Build history of the part. All positions in model axes, mm. Face numbers are marked on the shaded views. A direction names the side the tool comes from. Coordinates: 2 decimals unless noted, no trailing zeros. Order: outer loops, then holes, each group sorted by start corner. A loop starts at its lowest first (then second) coordinate and runs counter-clockwise, first axis right, second up. Notation, with made-up numbers: M -39.5,29.5 L 3.5,29.5 A26 ccw 3.5,65.5 Z; hole C -26,59 d8. An arc over 180 degrees is marked long. Write item = value, one per line. Start each with the question number.
Q1. Pull direction X, two halves, no side cores. Call the marked faces 1, 2 and 3: released by +X, released by -X, zero draft, split by the parting line, or undercut.
Q2. Pin check, flat tips, straight feed: P1, Ø6, axis at y = 21, z = -2.5, coming from the -X side; P2, Ø1.5, axis at x = -6, y = 21, coming from the -Z side; P3, Ø1, axis at x = -8.5, y = 16.5, coming from the +Z side. Stop position of each tip, or through.
Q3. Band-saw the part on A-A on y = 17.5. Write the cut outline in (x, z).
Q4. Drill centre lines: probe 1 along X at (y, z) = (1.3, 0); probe 2 along X at (y, z) = (20.25, 0); probe 3 along X at (y, z) = (11.5, 5). Where is each one in solid material? Low to high.
Q5. Band-saw the part on B-B on y = 6.5. Write the cut outline in (x, z).
Q6. 3-axis set-ups, long thin cutter, end or side, ignore diameter. For the marked faces 4 and 5: which of +Z, -Z, +X, -X, +Y, -Y reach the whole face in a straight line?
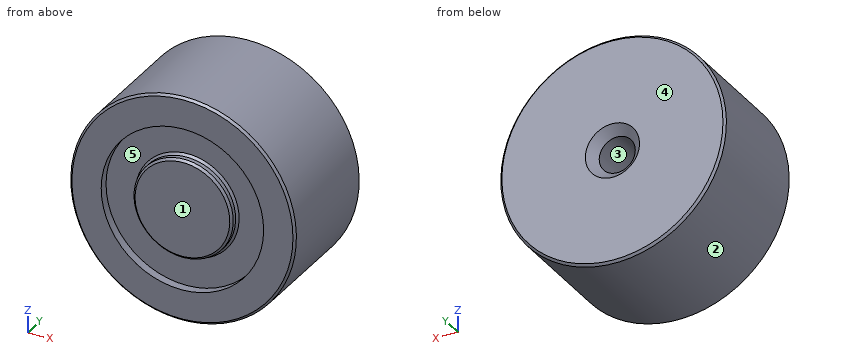
```python
from build123d import *

# Parameters (mm, degrees)
SKETCH_1_R          = 25
EXTRUDE_1_DEPTH     = 27
SKETCH_9_R          = 4
CUT_EXTRUDE_1_DEPTH = 12
CHAMFER_1_SIZE      = 2
CHAMFER_2_SIZE      = 0.5
SKETCH_11_R         = 18
SKETCH_11_R_2       = 11
CUT_EXTRUDE_2_DEPTH = 2
CHAMFER_3_SIZE      = 0.5


with BuildPart() as part:
    # 草图1 → 凸台-拉伸1 (new body)
    with BuildSketch(Plane(origin=(0, 0, 0), x_dir=(1, 0, 0), z_dir=(0, 1, 0))):
        with Locations(Location((0, 0, 0), (0, 0, 270))):
            Circle(SKETCH_1_R)
    extrude(amount=EXTRUDE_1_DEPTH)

    # 草图9 → 切除-拉伸1 (cut)
    with BuildSketch(Plane(origin=(0, 27, 0), x_dir=(1, 0, 0), z_dir=(0, 1, 0))):
        with Locations(Location((0, 0, 0), (0, 0, 270))):
            Circle(SKETCH_9_R)
    extrude(amount=-CUT_EXTRUDE_1_DEPTH, mode=Mode.SUBTRACT)

    # 草图10 → 切除-旋转2 (revolve, cut)
    with BuildSketch(Plane.XY, mode=Mode.PRIVATE) as cut_revolve_2_sk:
        Polygon((-4, 15), (0, 12.093829888), (0, 15), align=None)
    revolve(cut_revolve_2_sk.sketch.rotate(Axis((0, 12.093829888, 0), (0, 1, 0)), 90), axis=Axis((0, 12.093829888, 0), (0, 1, 0)), mode=Mode.SUBTRACT)

    # 倒角1
    chamfer_1_edges = [part.edges().sort_by_distance(p)[0] for p in [
        (0, 27, -4),
    ]]
    chamfer(chamfer_1_edges, length=CHAMFER_1_SIZE)

    # 倒角2
    chamfer_2_edges = [part.edges().sort_by_distance(p)[0] for p in [
        (0, 0, -25),
        (0, 27, -25),
    ]]
    chamfer(chamfer_2_edges, length=CHAMFER_2_SIZE)

    # 草图11 → 切除-拉伸2 (cut)
    with BuildSketch(Plane.XZ):
        with Locations(Location((0, 0, 0), (0, 0, 270))):
            Circle(SKETCH_11_R)
        with Locations(Location((0, 0, 0), (0, 0, 270))):
            Circle(SKETCH_11_R_2, mode=Mode.SUBTRACT)
    extrude(amount=-CUT_EXTRUDE_2_DEPTH, mode=Mode.SUBTRACT)

    # 倒角3
    chamfer_3_edges = [part.edges().sort_by_distance(p)[0] for p in [
        (0, 2, 11),
        (0, 0, 11),
    ]]
    chamfer(chamfer_3_edges, length=CHAMFER_3_SIZE)


solid = part.part
```
Recorded:
q1.face_1 = zero draft
q1.face_2 = split by the parting line
q1.face_3 = undercut
q2.P1 = -25
q2.P2 = -24.44
q2.P3 = 23.69
q3.outline = C 0,0 d50; hole C 0,0 d8
q4.probe_1 = -25 to -18, -11 to 11, 18 to 25
q4.probe_2 = -25 to -4, 4 to 25
q4.probe_3 = -24.49 to 24.49
q5.outline = C 0,0 d50
q6.face_4 = +Z, -Z, +X, -X, +Y
q6.face_5 = -Y
